Can you work these out from the model? Positions are in its coordinate system, mm. A direction names the side the tool comes from. Coordinates: 2 decimals unless noted, no trailing zeros. Order: outer loops, then holes, each group sorted by start corner. A loop starts at its lowest first (then second) coordinate and runs counter-clockwise, first axis right, second up. Notation, with made-up numbers: (44, -3) - (70, -3) arc R25 ccw to (70, 25) - close; hole circle Ø7 at (20.5, 22). An arc over 180 degrees is marked (long way). Return JSON: item names as keys, results as strings. Group by question number.
1) If we mould it in two halves opening along Y, with no side actions, what happens to faces 6 (the face through (0, 0, 1)), 7 (the face through (9, 10, 0)), 8 (the face through (-12, 8, 0)), 9 (the face through (0, 30, 0))? For each: pulls with the +Y half, pulls with the -Y half, needs draft (parallel to the pull), parting line crosses it, or undercut.
2) For pin 1 Ø10 at (x, y) = (7, 25) entering from +Z; pin 2 Ø2 at (x, y) = (8.5, 8) entering from +Z; pin 3 Ø0.9 at (y, z) = (24, 0) entering from -X; pin 4 Ø0.6 at (x, y) = (4.5, -1) entering from -Z, each with a flat end and sliding along its axis, tell me the tip position at first contact or that it passes through.
3) Imagine slicing it at D-D (z = 0.85). Write out the boundary of the cut face in (x, y), and give its area (3 significant figures).
4) Imagine slicing it at B-B (z = -0.95). Write out the boundary of the cut face in (x, y), and give its area (3 significant figures).
5) Which directions (+Z, -Z, +X, -X, +Y, -Y) give clear straight access to the entire face, cutting with the end or side of a thin tool? Please do faces 1 (the face through (0, 17, 1)), 2 (the face through (0, 28, 1)), 3 (the face through (11, 17, 0)), 4 (the face through (8.732, 5.542, -0.74)), 5 (the face through (-11, 17, 0)).
6) If I drill on line 1 along Y through (x, z) = (-3.25, 1.35); line 2 along X through (y, z) = (24, 0.7); line 3 along X through (y, z) = (10.5, 0.15), over which ranges is the centre line in solid material (lowest first)?
7) Imagine slicing it at C-C (y = 23). Write out the boundary of the cut face in (x, z), and give its area (3 significant figures).
8) Imagine slicing it at A-A (x = -3.75). Write out the boundary of the cut face in (y, z).
```python
from build123d import *

# Parameters (mm, degrees)
ESBO_O1_W                = 7.5
ESBO_O1_H                = 2
RESSALTO_EXTRUS_O1_DEPTH = 1.5
RESSALTO_EXTRUS_O2_DEPTH = 1.5


with BuildPart() as part:
    # Esbo_o1 → Ressalto-extrus_o1 (new body)
    with BuildSketch(Plane.XY):
        with Locations((3.75, 16)):
            Rectangle(ESBO_O1_W, ESBO_O1_H)
        with Locations((-3.75, 16)):
            Rectangle(ESBO_O1_W, ESBO_O1_H)
        Polygon((10, 2.5), (10, 0), (10, -2), (12, -2), (12, 17), (9.5, 17), (9.5, 30), (-9.5, 30), (-9.5, 17), (-12, 17), (-12, -2), (-10, -2), (-10, 0), (-10, 2.5), (-10, 15), (-7.5, 15), (-7.5, 17), (-7.5, 19.5), (-7.5, 28), (0, 28), (7.5, 28), (7.5, 19.5), (7.5, 17), (7.5, 15), (10, 15), (10, 8.5), align=None)
        Polygon((10, 0), (0, 0), (-10, 0), (-10, -2), (0, -2), (10, -2), align=None)
    extrude(amount=RESSALTO_EXTRUS_O1_DEPTH)

    # Esbo_o1_4 → Ressalto-extrus_o2 (add)
    with BuildSketch(Plane.XY):
        Polygon((10, 2.5), (10, -2), (12, -2), (12, 17), (9.5, 17), (9.5, 30), (-9.5, 30), (-9.5, 17), (-12, 17), (-12, -2), (-10, -2), (-10, 2.5), (-7.5, 8.5), (-7.5, 19.5), (7.5, 19.5), (7.5, 8.5), align=None)
    extrude(amount=-RESSALTO_EXTRUS_O2_DEPTH)


solid = part.part
```
Calculated:
{
 "1": {"face 6": "undercut", "face 7": "undercut", "face 8": "needs draft", "face 9": "pulls with the +Y half"},
 "2": {"pin 1": "z = 1.5", "pin 2": "z = 0", "pin 3": "x = -9.5", "pin 4": "z = 0"},
 "3": {"outline": "(-12, -2) - (12, -2) - (12, 17) - (9.5, 17) - (9.5, 30) - (-9.5, 30) - (-9.5, 17) - (-12, 17) - close; hole (-10, 0) - (10, 0) - (10, 15) - (-10, 15) - close; hole (-7.5, 17) - (7.5, 17) - (7.5, 28) - (-7.5, 28) - close", "area": "238 mm2"},
 "4": {"outline": "(-12, -2) - (-10, -2) - (-10, 2.5) - (-7.5, 8.5) - (-7.5, 19.5) - (7.5, 19.5) - (7.5, 8.5) - (10, 2.5) - (10, -2) - (12, -2) - (12, 17) - (9.5, 17) - (9.5, 30) - (-9.5, 30) - (-9.5, 17) - (-12, 17) - close", "area": "343 mm2"},
 "5": {"face 1": "+Z, -Z", "face 2": "+Z", "face 3": "+Z, -Z, +X, +Y", "face 4": "+Z, -Z, -Y", "face 5": "+Z, -Z, -X, +Y"},
 "6": {"line 1": "-2 to 0, 15 to 17, 28 to 30", "line 2": "-9.5 to -7.5, 7.5 to 9.5", "line 3": "-12 to -10, 10 to 12"},
 "7": {"outline": "(-9.5, -1.5) - (9.5, -1.5) - (9.5, 1.5) - (7.5, 1.5) - (7.5, 0) - (-7.5, 0) - (-7.5, 1.5) - (-9.5, 1.5) - close", "area": "34.5 mm2"},
 "8": {"outline": "(-2, 0) - (0, 0) - (0, 1.5) - (-2, 1.5) - close; (15, 0) - (17, 0) - (17, 1.5) - (15, 1.5) - close; (19.5, -1.5) - (30, -1.5) - (30, 1.5) - (28, 1.5) - (28, 0) - (19.5, 0) - close"}
}
